from build123d import *

# Parameters (mm, degrees)
F0_W     = 152.4
F0_H     = 254
F1_DEPTH = 9.525
F2_W     = 152.4
F2_H     = 254
F2_W_2   = 133.35
F2_H_2   = 234.95
F3_DEPTH = 57.15
F5_DEPTH = 152.401


with BuildPart() as f1:
    # F0 (on Top) → F1 (new body)
    with BuildSketch(Plane.XY):
        Rectangle(F0_W, F0_H)
    extrude(amount=F1_DEPTH)

    # F2 (on face) → F3 (join)
    with BuildSketch(Plane.XY.offset(9.525)):
        Rectangle(F2_W, F2_H)
        Rectangle(F2_W_2, F2_H_2, mode=Mode.SUBTRACT)
    extrude(amount=F3_DEPTH)

    # F4 (on face) → F5 (cut, through all)
    with BuildSketch(Plane.YZ.offset(76.2)):
        with BuildLine():
            Line((-127, 66.675), (-127, 19.05))
            Line((-127, 19.05), (-4.0201239704, 65.1674535111))
            add(Edge.make_bspline(
                [(-4.0201239704, 65.1674535111), (-4.084887365, 65.6563585182), (-4.1772574136, 66.1605990618), (-4.3000844307, 66.675)],
                knots=[0.9047570689, 0.9047570689, 0.9047570689, 0.9047570689, 1, 1, 1, 1], degree=3))
            Line((-4.3000844307, 66.675), (-127, 66.675))
        make_face()
        with BuildLine():
            Line((0, 66.675), (-4.0201239704, 65.1674535111))
            add(Edge.make_bspline(
                [(-6.35, 53.975), (-6.6047369801, 55.8170739007), (-5.1216855945, 58.6204590718), (-3.916212623, 61.1924199541), (-3.8355720634, 63.7742536647), (-4.0201239704, 65.1674535111)],
                knots=[0, 0, 0, 0, 0.3524232767, 0.6333496684, 0.9047570689, 0.9047570689, 0.9047570689, 0.9047570689], degree=3))
            ThreePointArc((-6.35, 53.975), (0, 60.325), (6.35, 53.975))
            add(Edge.make_bspline(
                [(6.35, 53.975), (6.6047369801, 55.8170739007), (5.1216855945, 58.6204590718), (3.7893136098, 61.4631678727), (3.8272454912, 64.6947451687), (4.3000844307, 66.675)],
                knots=[0, 0, 0, 0, 0.3524232767, 0.6333496684, 1, 1, 1, 1], degree=3))
            Line((4.3000844307, 66.675), (0, 66.675))
        make_face()
        with BuildLine():
            ThreePointArc((6.35, 53.975), (0, 60.325), (-6.35, 53.975))
            ThreePointArc((-6.35, 53.975), (0, 47.625), (6.35, 53.975))
        make_face()
        with BuildLine():
            add(Edge.make_bspline(
                [(-4.0201239704, 65.1674535111), (-4.084887365, 65.6563585182), (-4.1772574136, 66.1605990618), (-4.3000844307, 66.675)],
                knots=[0.9047570689, 0.9047570689, 0.9047570689, 0.9047570689, 1, 1, 1, 1], degree=3))
            Line((-4.0201239704, 65.1674535111), (0, 66.675))
            Line((0, 66.675), (-4.3000844307, 66.675))
        make_face()
    extrude(amount=-F5_DEPTH, mode=Mode.SUBTRACT)


solid = f1.part
Source: CAD feature listing. Evaluate the final solid. Frame: model axes, mm. A direction names the side the tool comes from. Round coordinates to 2 decimals unless told otherwise and drop trailing zeros. Order: outer loops, then holes, each group sorted by start corner. A loop starts at its lowest first (then second) coordinate and runs counter-clockwise, first axis right, second up. Notation, with made-up numbers: (21.25, 76.5) - (47.25, 76.5) arc R15 cw to (47.25, 80.5) - close; hole circle Ø8 at (-33, -40). An arc over 180 degrees is marked (long way). Use a Markdown table: item, result. Add a question column.
1. Section query C-C (x = 36). Return the cut outline in (y, z) (3 decimals).
2. Mould query, pull axis Z, two halves, no side actions, for faces 4 (the flat face through (-76.2, 26, 25)), 5 (the cylindrical face through (71.504, -0.14, 47.627)), 6 (the flat face through (-1, 2, 0)). Classes: +Z half, -Z half, draft (parallel to the pull), parting line (faces both ways), or undercut.
3. Set-up query: faces 1 (the flat face through (-1, -117.475, 16)), 2 (the cylindrical face through (-71.371, -0.14, 47.627)), 3 (the flat face through (-12, 120, 66.675)). Return all of +Z, -Z, +X, -X, +Y, -Y with unobstructed straight access to the full face (end or side cutting, diameter ignored); none if empty.
4. Section query A-A (y = -51). Return the cut outline in (x, z) (3 decimals), then the cut area to 3 significant figures.
5. Section query B-B (z = 12.5). Return the cut outline in (x, y) (3 decimals), then the cut area to 3 significant figures.
6. Line query: probe 1 along X at (y, z) = (5.5, 15.5) (3 decimals); probe 2 along Y at (x, z) = (-19, 14) (3 decimals); probe 3 along Z at (x, y) = (-27.5, 32.5) (3 decimals). Output: solid intervals per line, ascending.
7. First-contact query: pin 1 (12 mm diameter, centred on x = 41, y = 37.5, fed in from +Z) (3 decimals); pin 2 (1.5 mm diameter, centred on x = 23.5, z = 56.5, fed in from -Y) (3 decimals). Flat tips, straight axial feed; report the tip coordinate or a pass-through.
Derived:
| question | item | result |
|---|---|---|
| 1 | outline | (-127, 0) - (127, 0) - (127, 66.675) - (117.475, 66.675) - (117.475, 9.525) - (-117.475, 9.525) - (-117.475, 22.622) - (-127, 19.05) - close |
| 2 | face 4 | draft |
| 2 | face 5 | undercut |
| 2 | face 6 | -Z half |
| 3 | face 1 | +Z |
| 3 | face 2 | +X, -X |
| 3 | face 3 | +Z, +X, -X, +Y, -Y |
| 4 | outline | (-76.2, 0) - (76.2, 0) - (76.2, 47.55) - (66.675, 47.55) - (66.675, 9.525) - (-66.675, 9.525) - (-66.675, 47.55) - (-76.2, 47.55) - close |
| 4 | area | 2,180 mm2 |
| 5 | outline | (-76.2, -127) - (76.2, -127) - (76.2, 127) - (-76.2, 127) - close; hole (-66.675, -117.475) - (66.675, -117.475) - (66.675, 117.475) - (-66.675, 117.475) - close |
| 5 | area | 7,380 mm2 |
| 6 | probe 1 | -76.2 to -66.675, 66.675 to 76.2 |
| 6 | probe 2 | -127 to -117.475, 117.475 to 127 |
| 6 | probe 3 | 0 to 9.525 |
| 7 | pin 1 | z = 9.525 |
| 7 | pin 2 | y = 117.475 |
